For this review, use the dimensioned drawing (mm, ordinates from the lowest corner) and the shaded views. A direction names the side the tool comes from. Give positions to 0.01 mm unless a question says otherwise; leave off trailing zeros. Order: outer loops, then holes, each group sorted by start corner. A loop starts at its lowest first (then second) coordinate and runs counter-clockwise, first axis right, second up. Notation, with made-up numbers: (-21.75, 65.5) -> (11.25, 65.5) arc R15 cw to (11.25, 85.5) -> close; hole circle Ø11 at (55, -33). An arc over 180 degrees is marked (long way). Return JSON: item names as keys, results as strings.
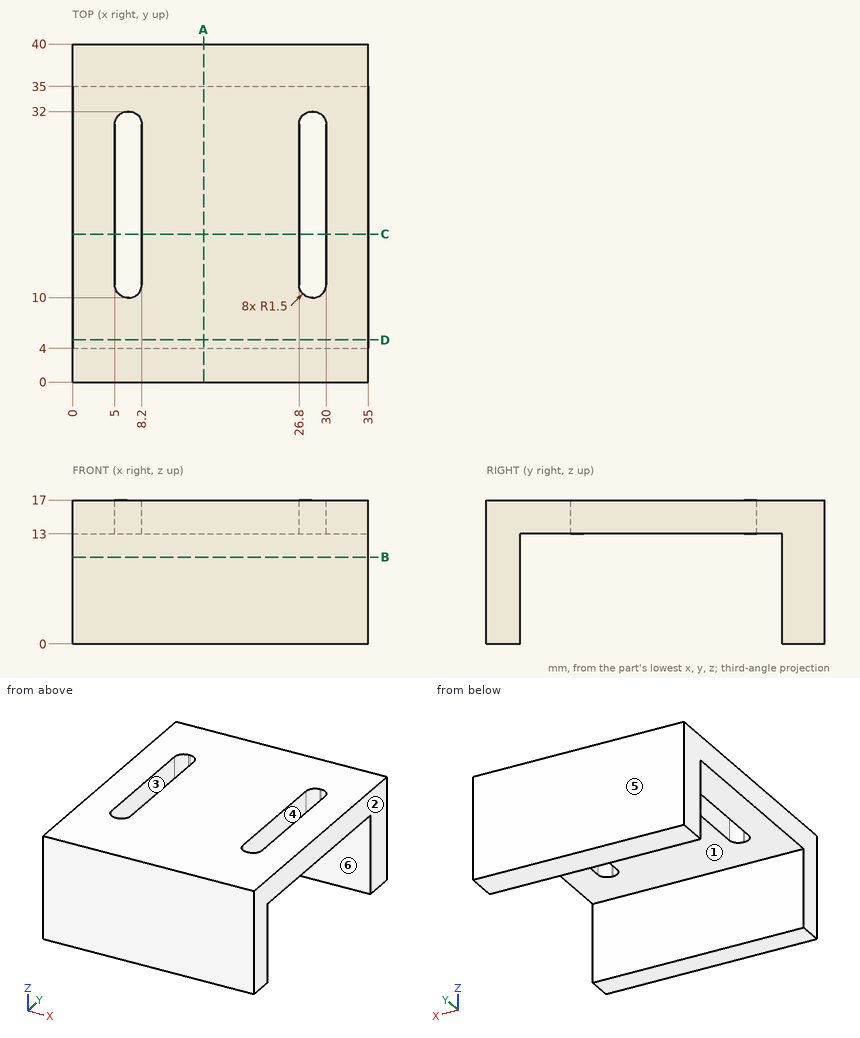
Item 1: Wall thickness on L1, parallel to X at y = 15.5, z = 13.75; L2, parallel to Y at x = 15.5, z = 12.75; L3, parallel to X at y = 31, z = 15.25: over which ranges is each line inside the solid? List them lowest first. Write a range as [from, to].
Result set:
{"L1": "x = [0, 5], [8.2, 26.8], [30, 35]", "L2": "y = [0, 4], [35, 40]", "L3": "x = [0, 5.09], [8.11, 26.89], [29.91, 35]"}
Item 2: Machinability: for the marked faces 5 and 6, which of the approach directions +Z, -Z, +X, -X, +Y, -Y give a long, thin tool a straight path to every point of the face, cutting with its end or side? Answer none if there is none.
Result set:
{"face 5": "+Z, -Z, +X, -X, +Y", "face 6": "-Z, +X, -X"}
Item 3: Add section B-B (z = 10.25). Give the boundary of the cut face in (x, y), plus the area to 3 significant figures.
Result set:
{"outline": "(0, 0) -> (35, 0) -> (35, 4) -> (0, 4) -> close; (0, 35) -> (35, 35) -> (35, 40) -> (0, 40) -> close", "area": "315 mm^2"}
Item 4: Add section C-C (y = 17.5). Give the boundary of the cut face in (x, z), plus the area to 3 significant figures.
Result set:
{"outline": "(0, 13) -> (5, 13) -> (5, 17) -> (0, 17) -> close; (8.2, 13) -> (26.8, 13) -> (26.8, 17) -> (8.2, 17) -> close; (30, 13) -> (35, 13) -> (35, 17) -> (30, 17) -> close", "area": "114 mm^2"}
Item 5: For pin 1 (5 mm diameter, centred on x = 11.5, y = 14.5, fed in from -Z), flat-tipped, find the tip position at first contact; note if it passes through.
Result set:
{"pin 1": "stops at z = 13"}
Item 6: Add section D-D (y = 5). Give the boundary of the cut face in (x, z).
Result set:
{"outline": "(0, 13) -> (35, 13) -> (35, 17) -> (0, 17) -> close"}
Item 7: Mouldability with a two-part tool opening along X and no side actions: class the marked faces 1, 2, 3 and 4 as released by +X, released by -X, zero draft, split by the parting line, or undercut.
Result set:
{"face 1": "zero draft", "face 2": "released by +X", "face 3": "undercut", "face 4": "undercut"}
Item 8: Add section A-A (x = 15.5). Give the boundary of the cut face in (y, z).
Result set:
{"outline": "(0, 0) -> (4, 0) -> (4, 13) -> (35, 13) -> (35, 0) -> (40, 0) -> (40, 17) -> (0, 17) -> close"}
